Verification items for this drawing (mm, ordinates from the low corner). Coordinates: 2 decimals unless noted, no trailing zeros. Write each loop counter-clockwise with the first axis right and the second up, starting at its lowest first coordinate (ties: lowest second). Pieces come first, ordered by that corner, then holes. Notation, with made-up numbers: M 60.25,38 L 107.25,38 A18 ccw 107.25,64 Z; hole C 77.5,30.5 d5. An arc over 180 degrees is marked long. Answer as CSV lines item,"result". Start each with the question number.
1) Section check D-D (y = 19). Record the cut outline in (x, z) (1 decimal).
2) Go/stop test with flat-tipped pins: pin 1 Ø3 at (x, z) = (129, 19) entering from +Y; pin 2 Ø1 at (x, z) = (75.5, 15) entering from -Y; pin 3 Ø2 at (x, z) = (26, 19.5) entering from -Y. Record where each tip stops, or that it passes through.
3) Section check A-A (y = 11). Record the cut outline in (x, z) (3 decimals), and give its area (3 significant figures).
4) Section check B-B (z = 11). Record the cut outline in (x, y) (1 decimal).
5) Draft check along Y on the marked faces 1 and 2. Enter one of: +Y half, -Y half, draft (parallel to the pull), parting line (faces both ways), or undercut.
6) Section check C-C (x = 10). Record the cut outline in (y, z), and give its area (3 significant figures).
7) Material ranges on L1, parallel to Y at x = 50, z = 11; L2, parallel to Y at x = 64.5, z = 7.5; L3, parallel to Z at x = 10, y = 1.4, recorded low to high. Write a range as [from, to].
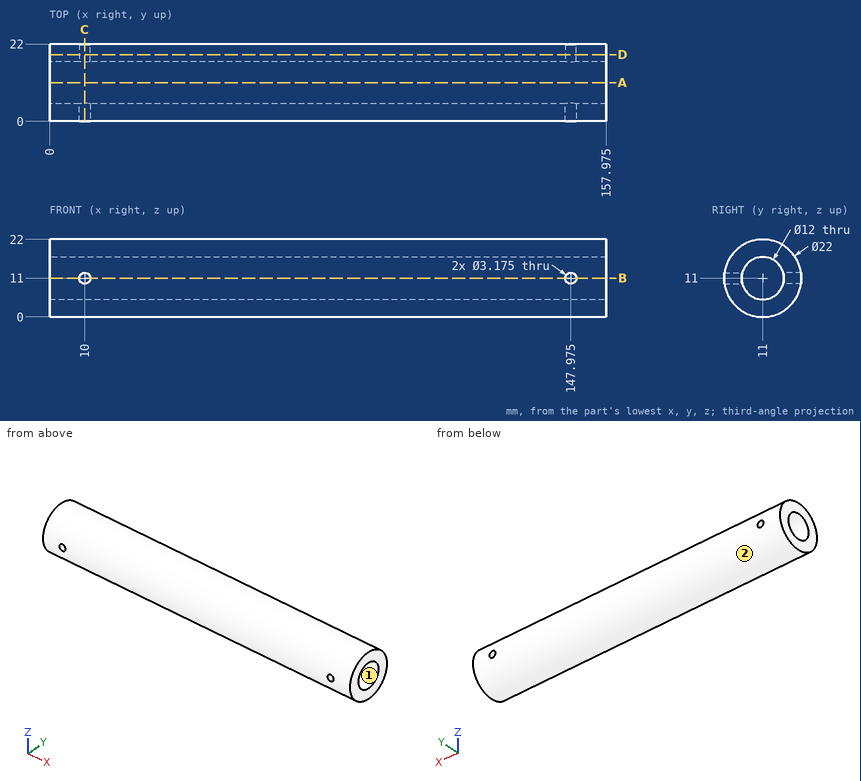
Results found:
1,outline,"M 0,3.5 L 158,3.5 L 158,18.5 L 0,18.5 Z; hole C 10,11 d3.2; hole C 148,11 d3.2"
2,pin 1,"stops at y = 19.87"
2,pin 2,"stops at y = 0.57"
2,pin 3,"stops at y = 2.95"
3,outline,"M 0,0 L 157.975,0 L 157.975,5 L 0,5 Z; M 0,17 L 157.975,17 L 157.975,22 L 0,22 Z"
3,area,"1,580 mm2"
4,outline,"M 0,0 L 8.4,0 L 8.4,5 L 0,5 Z; M 0,17 L 8.4,17 L 8.4,22 L 0,22 Z; M 11.6,0 L 146.4,0 L 146.4,5 L 11.6,5 Z; M 11.6,17 L 146.4,17 L 146.4,22 L 11.6,22 Z; M 149.6,0 L 158,0 L 158,5 L 149.6,5 Z; M 149.6,17 L 158,17 L 158,22 L 149.6,22 Z"
5,face 1,"undercut"
5,face 2,"parting line"
6,outline,"M 0.12,9.41 A11 ccw 21.88,9.41 L 16.79,9.41 A6 cw 5.21,9.41 Z; M 0.12,12.59 L 5.21,12.59 A6 cw 16.79,12.59 L 21.88,12.59 A11 ccw Z"
6,area,"235 mm2"
7,L1,"y = [0, 5], [17, 22]"
7,L2,"y = [0.57, 6.13], [15.87, 21.43]"
7,L3,"z = [5.63, 9.41], [12.59, 16.37]"
